The listing builds one solid part. Answer for the finished solid, in the listing's coordinates (mm). A direction names the side the tool comes from. Round coordinates to 2 decimals unless told otherwise and drop trailing zeros. Order: outer loops, then holes, each group sorted by start corner. A loop starts at its lowest first (then second) coordinate and runs counter-clockwise, first axis right, second up. Notation, with made-up numbers: (-3, 59) -> (30, 59) arc R24 ccw to (30, 75) -> close; hole circle Ø4 at (53.25, -22). An arc over 180 degrees is marked (long way). Return JSON: item names as keys, results as strings. Group by question number.
(1) The part is cut by section C-C (y = -125.5). Count the separate pieces of the cut face and the enclosed holes in it, plus the area to 3 significant figures.
(2) The part is cut by section B-B (z = 35.5). Determine the outline of the cut face in (x, y).
(3) Determine the mould class of faces 4 (the face through (-15, 130.5, -1)), 5 (the face through (2.6, -126, -66)), 6 (the face through (-15, -2, -70.5)) for opening direction Y: +Y half, -Y half, draft (parallel to the pull), parting line (faces both ways), or undercut.
(4) Consider line 1 (Z direction, x = 1, y = -125); line 2 (Y direction, x = 1, z = 65); line 3 (Y direction, x = -4, z = -34). Determine where each line is inside the solid, lowest interval first. Write a range as [from, to].
(5) The part is cut by section D-D (x = -4). Determine the outline of the cut face in (y, z).
(6) Each of these flat-tipped pins is pushed along its axis until it touches: pin 1 (4.5 mm diameter, centred on y = -7.5, z = -52.5, fed in from -X); pin 2 (6.5 mm diameter, centred on y = 7.5, z = -52.5, fed in from +X); pin 3 (5 mm diameter, centred on y = -125.5, z = 65.5, fed in from -X). Where does it stop, or does it pass through?
(7) Which of the six approach directions +Z, -Z, +X, -X, +Y, -Y give full straight-line access (tool end or side, diameter ignored) to faces 1 (the face through (1.479, -10.289, 49.804)), 2 (the face through (0.4, 126, -65)), 3 (the face through (-17, -121.2, -1))?
from build123d import *

# Parameters (mm, degrees)
SKETCH1_W                = 261
SKETCH1_H                = 141
SKETCH1_W_2              = 240
SKETCH1_H_2              = 120
SKETCH1_R                = 2
BOSS_EXTRUDE2_DEPTH      = 3
SKETCH1_6_W              = 261
SKETCH1_6_H              = 141
SKETCH1_6_W_2            = 240
SKETCH1_6_H_2            = 120
BOSS_EXTRUDE5_DEPTH      = 34
SKETCH14_W               = 259
SKETCH14_H               = 139
SKETCH14_W_2             = 258.2
SKETCH14_H_2             = 138.2
BOSS_EXTRUDE7_DEPTH      = 0.2
SKETCH17_W               = 259.4
SKETCH17_H               = 139.4
SKETCH17_W_2             = 258.2
SKETCH17_H_2             = 138.2
BOSS_EXTRUDE10_DEPTH     = 0.4
CHAMFER1_SIZE            = 0.4
CHAMFER1_SIZE_2          = 0.230940108
COVER_START              = -0.4
SKETCH18_R               = 3.15
COVER_MAGNET_HOLES_DEPTH = 2.2
SKETCH19_W               = 16
SKETCH19_H               = 240
CUT_EXTRUDE1_DEPTH       = 5
CHAMFER2_SIZE            = 3
CHAMFER2_SIZE_2          = 5.196152423
CHAMFER3_SIZE            = 5
CUT_EXTRUDE2_START       = -10.5
CUT_EXTRUDE2_DEPTH       = 11.5
CUT_EXTRUDE3_REACH       = 154.871
SKETCH21_W               = 242.4
SKETCH21_H               = 122.4


with BuildPart() as part:
    # Sketch1 → Boss-Extrude2 (new body)
    # profile 1 of 9: a face of its own
    with BuildSketch(Plane.YZ):
        Rectangle(SKETCH1_W, SKETCH1_H)
        Rectangle(SKETCH1_W_2, SKETCH1_H_2, mode=Mode.SUBTRACT)
    # profile 2 of 9: a face of its own
    with BuildSketch(Plane.YZ):
        with BuildLine():
            Line((-120, 60), (-120, 48))
            Line((-120, 48), (-114, 48))
            ThreePointArc((-114, 48), (-109.757359313, 49.757359313), (-108, 54))
            Line((-108, 54), (-108, 60))
            Line((-108, 60), (-120, 60))
        make_face()
        with Locations(Location((-112.5, 52.5, 0), (0, 0, 270))):
            Circle(SKETCH1_R, mode=Mode.SUBTRACT)
    # profile 3 of 9: a face of its own
    with BuildSketch(Plane.YZ):
        with BuildLine():
            Line((0, 60), (-12, 60))
            Line((-12, 60), (-12, 54))
            ThreePointArc((-12, 54), (-10.242640687, 49.757359313), (-6, 48))
            Line((-6, 48), (0, 48))
            Line((0, 48), (0, 60))
        make_face()
        with Locations(Location((-7.5, 52.5, 0), (0, 0, 270))):
            Circle(SKETCH1_R, mode=Mode.SUBTRACT)
    # profile 4 of 9: a face of its own
    with BuildSketch(Plane.YZ):
        with BuildLine():
            Line((12, 60), (0, 60))
            Line((0, 60), (0, 48))
            Line((0, 48), (6, 48))
            ThreePointArc((6, 48), (10.242640687, 49.757359313), (12, 54))
            Line((12, 54), (12, 60))
        make_face()
        with Locations(Location((7.5, 52.5, 0), (0, 0, 270))):
            Circle(SKETCH1_R, mode=Mode.SUBTRACT)
    # profile 5 of 9: a face of its own
    with BuildSketch(Plane.YZ):
        with BuildLine():
            Line((114, 48), (120, 48))
            Line((120, 48), (120, 60))
            Line((120, 60), (108, 60))
            Line((108, 60), (108, 54))
            ThreePointArc((108, 54), (109.757359313, 49.757359313), (114, 48))
        make_face()
        with Locations(Location((112.5, 52.5, 0), (0, 0, 270))):
            Circle(SKETCH1_R, mode=Mode.SUBTRACT)
    # profile 6 of 9: a face of its own
    with BuildSketch(Plane.YZ):
        with BuildLine():
            Line((108, -54), (108, -60))
            Line((108, -60), (120, -60))
            Line((120, -60), (120, -48))
            Line((120, -48), (114, -48))
            ThreePointArc((114, -48), (109.757359313, -49.757359313), (108, -54))
        make_face()
        with Locations(Location((112.5, -52.5, 0), (0, 0, 270))):
            Circle(SKETCH1_R, mode=Mode.SUBTRACT)
    # profile 7 of 9: a face of its own
    with BuildSketch(Plane.YZ):
        with BuildLine():
            Line((0, -48), (0, -60))
            Line((0, -60), (12, -60))
            Line((12, -60), (12, -54))
            ThreePointArc((12, -54), (10.242640687, -49.757359313), (6, -48))
            Line((6, -48), (0, -48))
        make_face()
        with Locations(Location((7.5, -52.5, 0), (0, 0, 270))):
            Circle(SKETCH1_R, mode=Mode.SUBTRACT)
    # profile 8 of 9: a face of its own
    with BuildSketch(Plane.YZ):
        with BuildLine():
            Line((-12, -54), (-12, -60))
            Line((-12, -60), (0, -60))
            Line((0, -60), (0, -48))
            Line((0, -48), (-6, -48))
            ThreePointArc((-6, -48), (-10.242640687, -49.757359313), (-12, -54))
        make_face()
        with Locations(Location((-7.5, -52.5, 0), (0, 0, 270))):
            Circle(SKETCH1_R, mode=Mode.SUBTRACT)
    # profile 9 of 9: a face of its own
    with BuildSketch(Plane.YZ):
        with BuildLine():
            Line((-120, -48), (-120, -60))
            Line((-120, -60), (-108, -60))
            Line((-108, -60), (-108, -54))
            ThreePointArc((-108, -54), (-109.757359313, -49.757359313), (-114, -48))
            Line((-114, -48), (-120, -48))
        make_face()
        with Locations(Location((-112.5, -52.5, 0), (0, 0, 270))):
            Circle(SKETCH1_R, mode=Mode.SUBTRACT)
    extrude(amount=BOSS_EXTRUDE2_DEPTH)

    # Sketch1<6> → Boss-Extrude5 (add)
    with BuildSketch(Plane.YZ):
        Rectangle(SKETCH1_6_W, SKETCH1_6_H)
        Rectangle(SKETCH1_6_W_2, SKETCH1_6_H_2, mode=Mode.SUBTRACT)
    extrude(amount=-BOSS_EXTRUDE5_DEPTH)

    # Sketch14 → Boss-Extrude7 (add)
    with BuildSketch(Plane(origin=(-34, 0, 0), x_dir=(0, -1, 0), z_dir=(-1, 0, 0))):
        Rectangle(SKETCH14_W, SKETCH14_H)
        Rectangle(SKETCH14_W_2, SKETCH14_H_2, mode=Mode.SUBTRACT)
    extrude(amount=BOSS_EXTRUDE7_DEPTH)

    # Sketch17 → Boss-Extrude10 (add)
    with BuildSketch(Plane(origin=(-34.2, 0, 0), x_dir=(0, -1, 0), z_dir=(-1, 0, 0))):
        Rectangle(SKETCH17_W, SKETCH17_H)
        Rectangle(SKETCH17_W_2, SKETCH17_H_2, mode=Mode.SUBTRACT)
    extrude(amount=BOSS_EXTRUDE10_DEPTH)

    # Chamfer1
    # the kernel refuses this chamfer: 0.4, 0.230940108 mm, written as the material it takes off along each edge
    with BuildSketch(Plane(origin=(-34.6, 130.734834302, -69.7), x_dir=(1, 0, 0), z_dir=(0, -1, 0))) as chamfer1_piece_1:
        Polygon((CHAMFER1_SIZE, 0), (0, CHAMFER1_SIZE_2 * 0.999999998596), (0, 0), align=None)
    extrude(amount=261.469668604, mode=Mode.SUBTRACT)
    with BuildSketch(Plane(origin=(-34.6, -129.7, -70.734834302), x_dir=(0, 1, 0), z_dir=(0, 0, 1)), Plane(origin=(-34.6, 129.7, 70.734834302), x_dir=(0, -1, 0), z_dir=(0, 0, -1))) as chamfer1_piece_2:
        Polygon((CHAMFER1_SIZE_2 * 0.999999998596, 0), (0, -CHAMFER1_SIZE), (0, 0), align=None)
    extrude(amount=141.469668604, mode=Mode.SUBTRACT)
    with BuildSketch(Plane(origin=(-34.6, -130.734834302, 69.7), x_dir=(0, 0, -1), z_dir=(0, 1, 0))) as chamfer1_piece_3:
        Polygon((CHAMFER1_SIZE_2 * 0.999999998596, 0), (0, -CHAMFER1_SIZE), (0, 0), align=None)
    extrude(amount=261.469668604, mode=Mode.SUBTRACT)

    # Sketch18 → Cover magnet holes (cut)
    with BuildSketch(Plane.YZ.offset(3).offset(COVER_START)):
        with Locations(Location((-125.5, 65.5, 0), (0, 0, 270))):
            Circle(SKETCH18_R)
        with Locations(Location((125.5, 65.5, 0), (0, 0, 90))):
            Circle(SKETCH18_R)
        with Locations(Location((125.5, -65.5, 0), (0, 0, 270))):
            Circle(SKETCH18_R)
        with Locations(Location((-125.5, -65.5, 0), (0, 0, 90))):
            Circle(SKETCH18_R)
    extrude(amount=-COVER_MAGNET_HOLES_DEPTH, mode=Mode.SUBTRACT)

    # Sketch19 → Cut-Extrude1 (cut)
    with BuildSketch(Plane(origin=(0, 0, 60), x_dir=(1, 0, 0), z_dir=(0, 0, -1))):
        with Locations((-21, 0)):
            Rectangle(SKETCH19_W, SKETCH19_H)
    extrude(amount=-CUT_EXTRUDE1_DEPTH, mode=Mode.SUBTRACT)

    # Chamfer2
    # the kernel refuses this chamfer: 5.196152423, 3 mm, written as the material it takes off along each edge
    with BuildSketch(Plane(origin=(-29, 120, 60), x_dir=(-1, 0, 0), z_dir=(0, -1, 0))) as chamfer2_piece_1_section:
        Polygon((CHAMFER2_SIZE, 0), (0, -CHAMFER2_SIZE_2), (0, 0), align=None)
    chamfer2_piece_1 = extrude(amount=240, mode=Mode.PRIVATE)
    chamfer2_piece_1 = split(chamfer2_piece_1, bisect_by=Plane(origin=(-29, 120, 65), z_dir=(0, 0, -1)), keep=Keep.TOP, mode=Mode.PRIVATE)
    add(chamfer2_piece_1, mode=Mode.SUBTRACT)

    # Chamfer3
    chamfer3_edges = [part.edges().sort_by_distance(p)[0] for p in [
        (-13, 0, 60),
    ]]
    chamfer(chamfer3_edges, length=CHAMFER3_SIZE - 0.0001)  # a hair under: the kernel refuses the full size

    # Cut-Extrude2: read off the stored shape, not the designer's step
    # Cut-Extrude2 outline → Cut-Extrude2 (cut)
    with BuildSketch(Plane(origin=(0, -120, 0), x_dir=(-1, 0, 0), z_dir=(0, 1, 0)).offset(CUT_EXTRUDE2_START)):
        Polygon((13, 65), (8, 60), (13, 55), (29.113248654, 55), (32, 60), (29.113248654, 65), align=None)
    extrude(amount=CUT_EXTRUDE2_DEPTH, mode=Mode.SUBTRACT)

    # Cut-Extrude3: up to this face of the body (flat: up to its plane)
    cut_extrude3_end = Plane(part.part.faces().sort_by_distance((0, 114.443379347, 54.443379347))[0])
    # Sketch21 → Cut-Extrude3 (cut, up to the picked face)
    with BuildSketch(Plane(origin=(-34, 0, 0), x_dir=(0, -1, 0), z_dir=(-1, 0, 0)), mode=Mode.PRIVATE) as cut_extrude3_sk1:
        Rectangle(SKETCH21_W, SKETCH21_H)
    cut_extrude3_tool1 = split(extrude(cut_extrude3_sk1.sketch, amount=-CUT_EXTRUDE3_REACH, mode=Mode.PRIVATE), bisect_by=cut_extrude3_end, keep=Keep.BOTH, mode=Mode.PRIVATE)
    add(cut_extrude3_tool1.solids().sort_by(Axis((-34, 0, 0), (1, 0, 0)))[0], mode=Mode.SUBTRACT)


solid = part.part
Answer below:
{
 "1": {"separate pieces": "1", "enclosed holes": "3", "area": "4,990 mm²"},
 "2": {"outline": "(-34.6, -129.47) -> (-34.2, -129.7) -> (-34.2, -129.5) -> (-34, -129.5) -> (-34, -130.5) -> (3, -130.5) -> (3, -120) -> (0, -120) -> (0, -121.2) -> (-34, -121.2) -> (-34, -129.1) -> (-34.6, -129.1) -> close; (-34.6, 129.1) -> (-34, 129.1) -> (-34, 121.2) -> (0, 121.2) -> (0, 120) -> (3, 120) -> (3, 130.5) -> (-34, 130.5) -> (-34, 129.5) -> (-34.2, 129.5) -> (-34.2, 129.7) -> (-34.6, 129.47) -> close"},
 "3": {"face 4": "+Y half", "face 5": "undercut", "face 6": "draft"},
 "4": {"line 1": "z = [-70.5, -68.61], [-62.39, 62.39], [68.61, 70.5]", "line 2": "y = [-130.5, -128.61], [-122.39, 122.39], [128.61, 130.5]", "line 3": "y = [-130.5, -121.2], [121.2, 130.5]"},
 "5": {"outline": "(-130.5, -70.5) -> (130.5, -70.5) -> (130.5, 70.5) -> (-130.5, 70.5) -> close; hole (-121.2, -61.2) -> (121.2, -61.2) -> (121.2, 61.2) -> (-121.2, 61.2) -> close"},
 "6": {"pin 1": "stops at x = 0", "pin 2": "stops at x = 3", "pin 3": "stops at x = -34"},
 "7": {"face 1": "+X, -X", "face 2": "none", "face 3": "-X"}
}
